```python
from build123d import *

# Parameters (mm, degrees)
F0_W      = 181
F0_H      = 76
F1_DEPTH  = 167
F2_W      = 25.2
F2_H      = 13
F3_DEPTH  = 39.4
F4_W      = 25.1968
F4_H      = 13.0048
F5_DEPTH  = 38.4
F6_W      = 2
F6_H      = 12
F7_DEPTH  = 11
F8_R      = 1
F9_R      = 2.75
F10_DEPTH = 3
F11_W     = 2
F11_H     = 11.9888
F12_DEPTH = 11
F13_R     = 1
F14_R     = 2.75
F15_DEPTH = 3
F16_R     = 3.6
F17_R     = 1


with BuildPart() as f1:
    # F0 (on Top) → F1 (new body)
    with BuildSketch(Plane.XY):
        with Locations((6.5742507577, -0.1865534149)):
            Rectangle(F0_W, F0_H)
    extrude(amount=F1_DEPTH)

    # F2 (on face) → F3 (cut)
    with BuildSketch(Plane.YZ.offset(97.0742507577)):
        with Locations((-25.5865534149, 160.5)):
            Rectangle(F2_W, F2_H)
    extrude(amount=-F3_DEPTH, mode=Mode.SUBTRACT)

    # F4 (on face) → F5 (cut)
    with BuildSketch(Plane(origin=(-83.9257492423, 0, 0), x_dir=(0, -1, 0), z_dir=(-1, 0, 0))):
        with Locations((25.5881534149, 160.4976)):
            Rectangle(F4_W, F4_H)
    extrude(amount=-F5_DEPTH, mode=Mode.SUBTRACT)

    # F6 (on face) → F7 (join)
    with BuildSketch(Plane.XY.offset(154)):
        with Locations((73.2742507577, -24.9865534149)):
            Rectangle(F6_W, F6_H)
    extrude(amount=F7_DEPTH)

    # F8
    f8_edges = [f1.edges().sort_by_distance(p)[0] for p in [
        (73.274251, -30.986553, 165),
        (73.274251, -18.986553, 165),
    ]]
    fillet(f8_edges, radius=F8_R)

    # F9 (on face) → F10 (cut)
    with BuildSketch(Plane.YZ.offset(74.2742507577)):
        with Locations((-24.9865534149, 160)):
            Circle(F9_R)
    extrude(amount=-F10_DEPTH, mode=Mode.SUBTRACT)

    # F11 (on face) → F12 (join)
    with BuildSketch(Plane.XY.offset(153.9952)):
        with Locations((-60.1165492423, -25.0039534149)):
            Rectangle(F11_W, F11_H)
    extrude(amount=F12_DEPTH)

    # F13
    f13_edges = [f1.edges().sort_by_distance(p)[0] for p in [
        (-60.116549, -30.998353, 164.9952),
        (-60.116549, -19.009553, 164.9952),
    ]]
    fillet(f13_edges, radius=F13_R)

    # F14 (on face) → F15 (cut)
    with BuildSketch(Plane(origin=(-61.1165492423, 0, 0), x_dir=(0, -1, 0), z_dir=(-1, 0, 0))):
        with Locations((25.0039534149, 159.9952)):
            Circle(F14_R)
    extrude(amount=-F15_DEPTH, mode=Mode.SUBTRACT)

    # F16
    f16_edges = [f1.edges().sort_by_distance(p)[0] for p in [
        (97.074251, -38.186553, 77),
        (97.074251, -0.186553, 0),
        (97.074251, 37.813447, 83.5),
        (6.574251, 37.813447, 0),
        (6.574251, -38.186553, 0),
        (-83.925749, 37.813447, 83.5),
        (-83.925749, -0.186553, 0),
        (-83.925749, -38.186553, 76.9976),
    ]]
    fillet(f16_edges, radius=F16_R)

    # F17
    f17_edges = [f1.edges().sort_by_distance(p)[0] for p in [
        (-62.925749, -38.186553, 153.9952),
        (-83.925749, -23.788153, 153.9952),
        (-83.925749, -12.989753, 160.4976),
        (-64.725749, -12.989753, 167),
        (-45.525749, -25.588153, 167),
        (-45.525749, -12.989753, 160.4976),
        (-45.525749, -25.588153, 153.9952),
        (-64.725749, -12.989753, 153.9952),
        (-45.525749, -38.186553, 160.4976),
        (6.074251, -38.186553, 167),
        (-83.925749, 10.611847, 167),
        (77.374251, -12.986553, 167),
        (57.674251, -25.586553, 167),
        (57.674251, -12.986553, 160.5),
        (77.374251, -12.986553, 154),
        (57.674251, -25.586553, 154),
        (57.674251, -38.186553, 160.5),
        (75.574251, -38.186553, 154),
        (97.074251, -12.986553, 160.5),
        (97.074251, -23.786553, 154),
    ]]
    fillet(f17_edges, radius=F17_R)


solid = f1.part
```
Input: part model. Units: mm. Frame: model coordinates. A direction names the side the tool comes from. Round coordinates to 2 decimals unless told otherwise and drop trailing zeros. Loops run counter-clockwise (first coordinate to the right, second up) from the corner with the lowest first, then second, coordinate; pieces in that order, holes last. Notation, with made-up numbers: (27.25, -30) -> (70.25, -30) arc R15 cw to (70.25, -3) -> close; hole circle Ø2 at (33.25, -13.75). An arc over 180 degrees is marked (long way). Use one line per item in the form item = value. Start each with the question number.
Item 1: Contact query for flat-ended pins moving along their axis: pin 1 Ø1.6 at (x, z) = (73.5, 157.5) entering from -Y; pin 2 Ø1 at (x, y) = (73, -23.5) entering from +Z; pin 3 Ø9 at (y, z) = (-25.5, 159) entering from -X. Output: stop coordinate, or through.
Item 2: Material intervals for L1, parallel to Y at x = 73.5, z = 160; L2, parallel to Z at x = -74.5, y = -29; L3, parallel to Y at x = 72, z = 160, sorted ascending. Write a range as from..to.
Item 3: Mould query, pull axis X, two halves, no side actions, for faces 6 (the face through (78, -26, 154)), 7 (the face through (-45.526, -25, 161)), 8 (the face through (5, 37.813, 84)), 9 (the face through (74.274, -25, 157)). Classes: pulls with the +X half, pulls with the -X half, needs draft (parallel to the pull), parting line crosses it, or undercut.
Item 4: Section query A-A on x = -54. Return the cut outline in (y, z).
Item 5: Set-up query: faces 1 (the face through (-60.131, -24.646, 162.722)), 2 (the face through (57.674, -26, 161)), 3 (the face through (73.29, -23.72, 157.56)), 4 (the face through (-61.117, -25, 157)), 5 (the face through (5, 9, 167)). Return all of +Z, -Z, +X, -X, +Y, -Y with unobstructed straight access to the full face (end or side cutting, diameter ignored); none if empty.
Ans:
q1.pin_1 = -30.99
q1.pin_2 = 165
q1.pin_3 = -61.12
q2.L1 = -30.99..-27.74, -22.24..-18.99, -12.99..37.81
q2.L2 = 0..154
q2.L3 = -12.99..37.81
q3.face_6 = undercut
q3.face_7 = undercut
q3.face_8 = needs draft
q3.face_9 = pulls with the +X half
q4.outline = (-38.19, 3.6) arc R3.6 ccw to (-34.59, 0) -> (34.21, 0) arc R3.6 ccw to (37.81, 3.6) -> (37.81, 166) arc R1 ccw to (36.81, 167) -> (-11.99, 167) arc R1 ccw to (-12.99, 166) -> (-12.99, 155) arc R1 cw to (-13.99, 154) -> (-37.19, 154) arc R1 ccw to (-38.19, 153) -> close
q5.face_1 = -X
q5.face_2 = +Z, -Y
q5.face_3 = +X
q5.face_4 = +Z, -X, -Y
q5.face_5 = +Z, +X, -X, +Y, -Y
